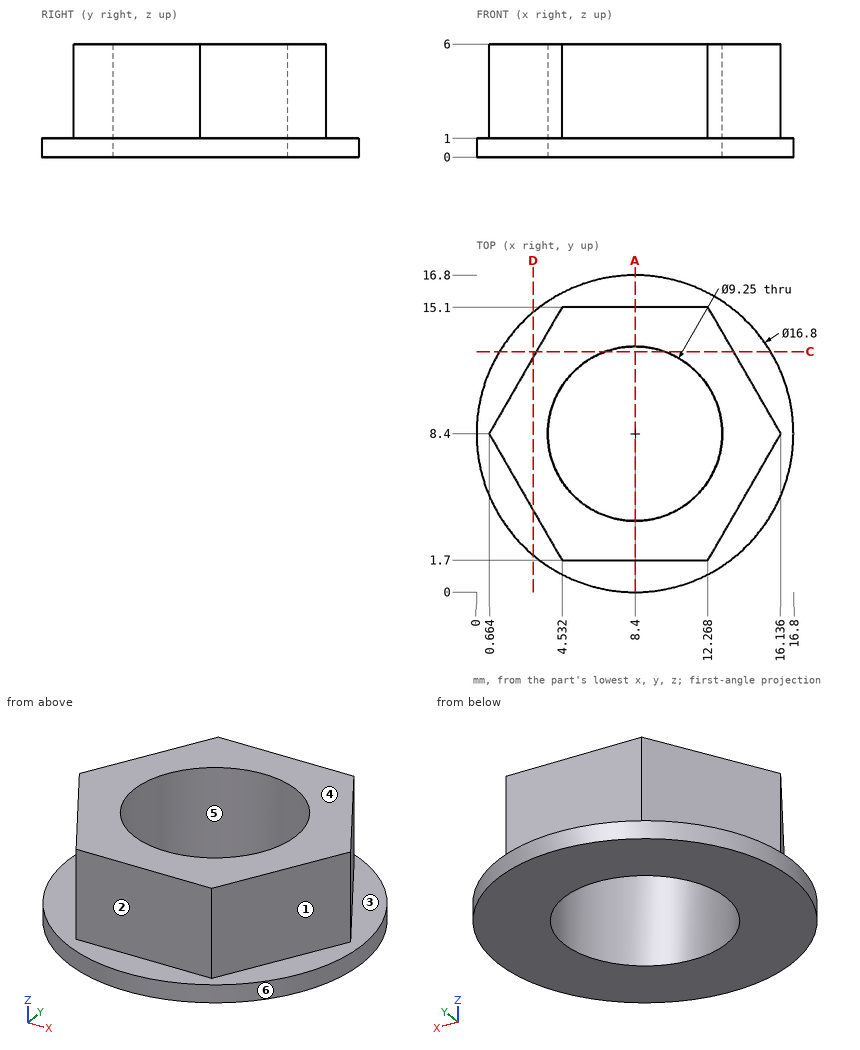
Answer from the drawing. Dimensions are ordinates in mm from the lowest x, y and z of the part. A direction names the side the tool comes from. Round coordinates to 2 decimals unless told otherwise and drop trailing zeros. Write each loop counter-clockwise with the first axis right and the second up, starting at its lowest first coordinate (ties: lowest second). Pieces come first, ordered by that corner, then holes. Notation, with made-up numbers: M 55.25,-8 L 98.25,-8 A31 ccw 98.25,28 Z; hole C 70,87.5 d8. An arc over 180 degrees is marked long. Write each question's results on one line, items separated by ' | '. Start each with the question number.
Item 1: Find section A-A on x = 8.4. Write down the section's boundary in (y, z) (1 decimal).
Item 2: The mould has two halves that part along X. Classify the marked faces 4, 5 and 6: +X half, -X half, draft (parallel to the pull), parting line (faces both ways), or undercut.
Item 3: Given pin 1 Ø1.5 at (x, z) = (10, 2.5) entering from +Y; pin 2 Ø8.5 at (x, y) = (8.4, 8.4) entering from -Z; pin 3 Ø1.5 at (y, z) = (10.5, 2) entering from -X; pin 4 Ø1.5 at (x, z) = (9.5, 3) entering from -Y, each flat-ended and moving along its own axis, determine where each tip first touches the part or whether it passes through.
Item 4: Straight lines are drawn through the part: probe 1 along Y at (x, z) = (8.4, 2.85) (1 decimal); probe 2 along X at (y, z) = (10.5, 4.95) (1 decimal); probe 3 along X at (y, z) = (8.25, 2.3). For each, find the intervals that lie inside material, in ascending order.
Item 5: Find section D-D on x = 3. Write down the section's boundary in (y, z) (1 decimal).
Item 6: Which of the six approach directions +Z, -Z, +X, -X, +Y, -Y give full straight-line access (tool end or side, diameter ignored) to the marked faces 1, 2 and 3?
Item 7: Find section C-C on y = 12.75. Write down the section's boundary in (x, z) (1 decimal).
Answer block:
1) outline: M 0,0 L 3.8,0 L 3.8,6 L 1.7,6 L 1.7,1 L 0,1 Z; M 13,0 L 16.8,0 L 16.8,1 L 15.1,1 L 15.1,6 L 13,6 Z
2) face 4: draft | face 5: undercut | face 6: parting line
3) pin 1: stops at y = 15.1 | pin 2: passes through | pin 3: stops at x = 1.44 | pin 4: stops at y = 1.7
4) probe 1: y = 1.7 to 3.8, 13 to 15.1 | probe 2: x = 1.9 to 4.3, 12.5 to 14.9 | probe 3: x = 0.75 to 3.78, 13.02 to 16.05
5) outline: M 2,0 L 14.8,0 L 14.8,1 L 12.4,1 L 12.4,6 L 4.4,6 L 4.4,1 L 2,1 Z
6) face 1: +Z, +X, -Y | face 2: +Z, +X, -X, -Y | face 3: +Z
7) outline: M 1.2,0 L 6.8,0 L 6.8,6 L 3.2,6 L 3.2,1 L 1.2,1 Z; M 10,0 L 15.6,0 L 15.6,1 L 13.6,1 L 13.6,6 L 10,6 Z
